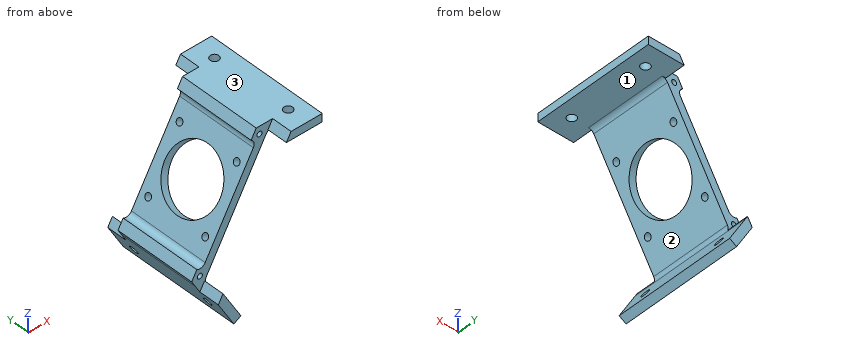
from build123d import *

# Parameters (mm, degrees)
BOSS_EXTRUDE4_DEPTH = 60
CUT_EXTRUDE9_DEPTH  = 10
FILLET5_R           = 3
SKETCH13_R          = 1.25
CUT_EXTRUDE10_DEPTH = 51
SKETCH14_R          = 2.125
CUT_EXTRUDE11_DEPTH = 4
SKETCH15_R          = 2.125
CUT_EXTRUDE12_DEPTH = 4
SKETCH16_R          = 15
SKETCH16_R_2        = 1.6
CUT_EXTRUDE13_DEPTH = 4
CUT_EXTRUDE14_DEPTH = 40


with BuildPart() as part:
    # Sketch1 → Boss-Extrude4 (new body)
    with BuildSketch(Plane(origin=(0, 0, 0), x_dir=(1, 0, 0), z_dir=(0, 1, 0))):
        with BuildLine():
            Line((84.5, 10), (104.5, 10))
            Line((104.5, 10), (104.5, 14))
            Line((104.5, 14), (88.541451884, 14))
            ThreePointArc((88.541451884, 14), (87.041451884, 14.401923789), (85.943375673, 15.5))
            Line((85.943375673, 15.5), (56.395081595, 66.67914662))
            ThreePointArc((56.395081595, 66.67914662), (55.993157806, 68.17914662), (56.395081595, 69.67914662))
            Line((56.395081595, 69.67914662), (64.374355653, 83.499654695))
            Line((64.374355653, 83.499654695), (60.910254038, 85.499654695))
            Line((60.910254038, 85.499654695), (50.910254038, 68.17914662))
            Line((50.910254038, 68.17914662), (46.868804038, 61.179149884))
            Line((46.868804038, 61.179149884), (49.178205115, 57.179149884))
            Line((49.178205115, 57.179149884), (53.219655115, 64.17914662))
            Line((53.219655115, 64.17914662), (82.190598923, 14))
            Line((82.190598923, 14), (74.107698923, 14))
            Line((74.107698923, 14), (76.4171, 10))
            Line((76.4171, 10), (84.5, 10))
        make_face()
    extrude(amount=BOSS_EXTRUDE4_DEPTH)

    # Sketch12 → Cut-Extrude9 (cut)
    with BuildSketch(Plane(origin=(0, 60, 0), x_dir=(1, 0, 0), z_dir=(0, 1, 0))):
        with BuildLine():
            Line((89.118802154, 10), (76.4171, 10))
            Line((76.4171, 10), (46.868804038, 61.179149884))
            Line((46.868804038, 61.179149884), (53.219655115, 72.17914662))
            Line((53.219655115, 72.17914662), (55.529056191, 68.17914662))
            Line((55.529056191, 68.17914662), (56.395081595, 69.67914662))
            ThreePointArc((56.395081595, 69.67914662), (55.993157806, 68.17914662), (56.395081595, 66.67914662))
            Line((56.395081595, 66.67914662), (85.943375673, 15.5))
            ThreePointArc((85.943375673, 15.5), (87.041451884, 14.401923789), (88.541451884, 14))
            Line((88.541451884, 14), (86.809401077, 14))
            Line((86.809401077, 14), (89.118802154, 10))
        make_face()
    cut_extrude9 = extrude(amount=-CUT_EXTRUDE9_DEPTH, mode=Mode.SUBTRACT)

    # Mirror4: Cut-Extrude9 across plane
    add(cut_extrude9.mirror(Plane.ZX.offset(30)), mode=Mode.SUBTRACT)

    # Fillet5
    fillet5_edges = [part.edges().sort_by_distance(p)[0] for p in [
        (82.190598923, 30, -14),
        (53.219655115, 30, -64.17914662),
    ]]
    fillet(fillet5_edges, radius=FILLET5_R)

    # Sketch13 → Cut-Extrude10 (cut, through all)
    with BuildSketch(Plane(origin=(0, 50, 0), x_dir=(1, 0, 0), z_dir=(0, 1, 0))):
        with Locations((53.2197, 64.6791)):
            Circle(SKETCH13_R)
        with Locations((82.6236, 13.75)):
            Circle(SKETCH13_R)
    extrude(amount=-CUT_EXTRUDE10_DEPTH, mode=Mode.SUBTRACT)

    # Sketch14 → Cut-Extrude11 (cut)
    with BuildSketch(Plane.XY.offset(-10)):
        with Locations((96.809401077, 50)):
            Circle(SKETCH14_R)
        with Locations((96.809401077, 10)):
            Circle(SKETCH14_R)
    extrude(amount=-CUT_EXTRUDE11_DEPTH, mode=Mode.SUBTRACT)

    # Sketch15 → Cut-Extrude12 (cut)
    with BuildSketch(Plane(origin=(8.660254038, 0, 5), x_dir=(-0.5, 0, 0.866025404), z_dir=(-0.866025404, 0, -0.5))):
        with Locations((-96.809401077, 50)):
            Circle(SKETCH15_R)
        with Locations((-96.809401077, 10)):
            Circle(SKETCH15_R)
    extrude(amount=-CUT_EXTRUDE12_DEPTH, mode=Mode.SUBTRACT)

    # Sketch16 → Cut-Extrude13 (cut)
    with BuildSketch(Plane(origin=(71.169228634, 0, -41.08957331), x_dir=(-0.5, 0, -0.866025404), z_dir=(0.866025404, 0, -0.5))):
        with Locations((0, 30)):
            Circle(SKETCH16_R)
        with Locations((-15.5, 45.5)):
            Circle(SKETCH16_R_2)
        with Locations((15.5, 45.5)):
            Circle(SKETCH16_R_2)
        with Locations((15.5, 14.5)):
            Circle(SKETCH16_R_2)
        with Locations((-15.5, 14.5)):
            Circle(SKETCH16_R_2)
    extrude(amount=-CUT_EXTRUDE13_DEPTH, mode=Mode.SUBTRACT)

    # Sketch17 → Cut-Extrude14 (cut)
    with BuildSketch(Plane(origin=(0, 50, 0), x_dir=(1, 0, 0), z_dir=(0, 1, 0))):
        Polygon((46.868804038, 61.179149884), (76.4171, 10), (81.0358, 10), (49.178154038, 65.179061416), align=None)
    extrude(amount=-CUT_EXTRUDE14_DEPTH, mode=Mode.SUBTRACT)


solid = part.part
Could you check a few things on this model? Use its own coordinates, in mm. Face numbers are marked on the shaded views. Give positions to 0.01 mm unless a question says otherwise; leave off trailing zeros. Order: outer loops, then holes, each group sorted by start corner. A loop starts at its lowest first (then second) coordinate and runs counter-clockwise, first axis right, second up. Notation, with made-up numbers: (-28.5, -1) -> (8.5, -1) arc R8 cw to (8.5, 11) -> close; hole circle Ø5 at (78, 52.5). An arc over 180 degrees is marked (long way). Return JSON: item names as keys, results as strings.
1. Imagine slicing it at A-A on y = 19. List the corners of the cut face in (x, z) for me, then the cut area to 3 significant figures.
Answer list:
{"outline": "(49.18, -65.18) -> (60.91, -85.5) -> (64.37, -83.5) -> (56.4, -69.68) arc R3 cw to (56.4, -66.68) -> (66.07, -49.92) -> (62.61, -47.92) -> (55.82, -59.68) arc R3 cw to (51.72, -60.78) -> close; (72.8, -30.26) -> (76.27, -32.26) -> (85.94, -15.5) arc R3 cw to (88.54, -14) -> (104.5, -14) -> (104.5, -10) -> (81.04, -10) -> (78.49, -14.4) arc R3 cw to (79.59, -18.5) -> close; hole circle Ø2.5 at (53.22, -64.68); hole circle Ø2.5 at (82.62, -13.75)", "area": "359 mm2"}
2. Imagine slicing it at D-D on z = -73.5. List the corners of the cut face in (x, y) for me.
Answer list:
{"outline": "(53.98, 0) -> (58.6, 0) -> (58.6, 60) -> (53.98, 60) -> close"}
3. I need wall thicknesses on line 1 (Z direction, x = 91, y = 17.5); line 2 (Z direction, x = 63.5, y = 19); line 3 (X direction, y = 36, z = -60.5). Which ranges of each line are inside material? Lowest first, please. Write a range as from..to.
Answer list:
{"line 1": "z = -14..-10", "line 2": "z = -84..-81.99, -54.37..-48.44", "line 3": "x = 55.12..59.96"}
4. Imagine slicing it at C-C on x = 101.5. List the corners of the cut face in (y, z) for me.
Answer list:
{"outline": "(0, -14) -> (60, -14) -> (60, -10) -> (0, -10) -> close"}
5. Thinking about a two-plate mould opening in Z: for the marked faces 1, 2 and 3, which applies, pulls with the +Z half, pulls with the -Z half, needs draft (parallel to the pull), parting line crosses it, or undercut?
Answer list:
{"face 1": "pulls with the -Z half", "face 2": "undercut", "face 3": "pulls with the +Z half"}
6. For pin 1 Ø10 at (y, z) = (36.5, -19.5) entering from +X; pin 2 Ø1.5 at (x, y) = (99, 25.5) entering from -Z; pin 3 Ø1 at (x, y) = (58.5, 50.5) entering from -Z; pin 4 Ø3.5 at (x, y) = (96.81, 50) entering from -Z, each with a flat end and sliding along its axis, tell me the tip position at first contact or that it passes through.
Answer list:
{"pin 1": "stops at x = 86.88", "pin 2": "stops at z = -14", "pin 3": "stops at z = -82.19", "pin 4": "passes through"}
7. Imagine slicing it at B-B on y = 26.5. List the corners of the cut face in (x, z) for me.
Answer list:
{"outline": "(49.18, -65.18) -> (60.91, -85.5) -> (64.37, -83.5) -> (56.4, -69.68) arc R3 cw to (56.4, -66.68) -> (63.88, -53.72) -> (60.41, -51.72) -> (55.82, -59.68) arc R3 cw to (51.72, -60.78) -> close; (75, -26.46) -> (78.46, -28.46) -> (85.94, -15.5) arc R3 cw to (88.54, -14) -> (104.5, -14) -> (104.5, -10) -> (81.04, -10) -> (78.49, -14.4) arc R3 cw to (79.59, -18.5) -> close; hole circle Ø2.5 at (53.22, -64.68); hole circle Ø2.5 at (82.62, -13.75)"}
